For this review, take the finished solid that the model builds, in its own axes (mm). Face numbers are marked on the shaded views. A direction names the side the tool comes from. Round coordinates to 2 decimals unless told otherwise and drop trailing zeros. Write each loop counter-clockwise with the first axis right and the second up, starting at its lowest first coordinate (ties: lowest second). Pieces come first, ordered by that corner, then holes. Notation, with made-up numbers: (46.5, -32.5) -> (67.5, -32.5) arc R4 cw to (67.5, -26.5) -> close; hole circle Ø9 at (9.25, -33.75). An arc over 180 degrees is marked (long way). Write each question's results on one line, items separated by ' | '. Start each with the question number.
Item 1: Tool access review of the marked faces 1, 2, 3 and 4: name each direction out of +Z, -Z, +X, -X, +Y, -Y from which nothing blocks a thin tool from reaching the whole face with its end or side.
Item 2: The part is to be moulded in two halves that separate along X. For the marked faces 5, 6 and 7, say which applies: +X half, -X half, draft (parallel to the pull), parting line (faces both ways), or undercut.
Item 3: To check wall thickness, follow line 1 along Z through (x, y) = (2, 20.25); line 2 along Y through (x, z) = (0, 0.3); line 3 along Y through (x, z) = (-4.25, 2). State the ranges of each line that lie inside material, in increasing order.
Item 4: Add section C-C (x = 4). State the section outline as (y, z) points.
Item 5: Add section B-B (z = -4). State the section outline as (x, y) points, plus the area to 3 significant figures.
Item 6: Clearance check with flat-ended pins moving along their axes: pin 1 (4 mm diameter, centred on y = 21.5, z = 0, fed in from -X); pin 2 (1 mm diameter, centred on x = 2.5, y = 20, fed in from -Z); pin 3 (0.8 mm diameter, centred on x = -2, y = 6, fed in from -Z); pin 4 (2 mm diameter, centred on x = 2, z = 1, fed in from -Y). State where each tip first meets the part, or that it passes through.
Item 7: Add section A-A (y = 22). State the section outline as (x, z) points.
from build123d import *

# Parameters (mm, degrees)
SKETCH3_R           = 4.65
BOSS_EXTRUDE1_DEPTH = 20
SKETCH4_R           = 1
BOSS_EXTRUDE2_DEPTH = 2.5
BOSS_EXTRUDE3_START = -2.5
BOSS_EXTRUDE3_DEPTH = 10
CIRPATTERN1_COUNT   = 4
CIRPATTERN1_ANGLE   = 45


with BuildPart() as part:
    # Sketch3 → Boss-Extrude1 (new body)
    with BuildSketch(Plane(origin=(0, 0, 0), x_dir=(1, 0, 0), z_dir=(0, 1, 0))):
        with Locations(Location((0, 0, 0), (0, 0, 270))):
            Circle(SKETCH3_R)
    extrude(amount=BOSS_EXTRUDE1_DEPTH)

    # Sketch4 → Boss-Extrude2 (add, symmetric)
    with BuildSketch(Plane.XY):
        with BuildLine():
            Line((3, 20), (-3, 20))
            Line((-3, 20), (-3, 25))
            ThreePointArc((-3, 25), (0, 28), (3, 25))
            Line((3, 25), (3, 20))
        make_face()
        with Locations((0, 25)):
            Circle(SKETCH4_R, mode=Mode.SUBTRACT)
    extrude(amount=BOSS_EXTRUDE2_DEPTH, both=True)

    # Sketch5 → Boss-Extrude3 (add)
    with BuildSketch(Plane.XZ.offset(BOSS_EXTRUDE3_START)):
        Polygon((-5, 0), (-2.5, -4.330127019), (2.5, -4.330127019), (5, 0), (2.5, 4.330127019), (-2.5, 4.330127019), align=None)
    boss_extrude3 = extrude(amount=-BOSS_EXTRUDE3_DEPTH)

    # CirPattern1: Boss-Extrude3 ×4 about axis
    cirpattern1_axis = Axis((0, 0, 0), (0, -1, 0))
    for i in range(1, CIRPATTERN1_COUNT):
        add(boss_extrude3.rotate(cirpattern1_axis, i * CIRPATTERN1_ANGLE / (CIRPATTERN1_COUNT - 1)))


solid = part.part
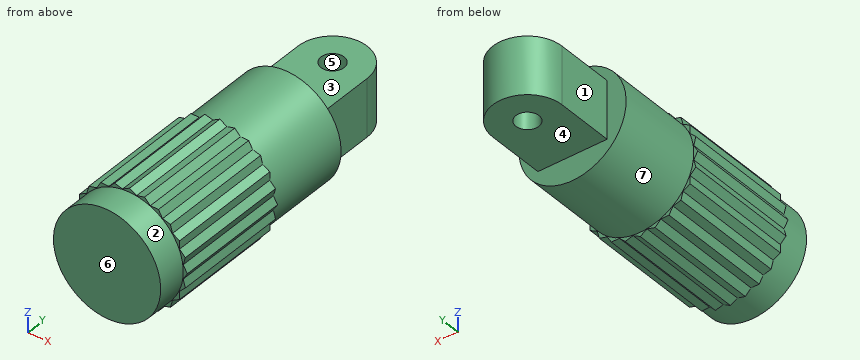
Responses:
1) face 1: +Z, -Z, -X, +Y | face 2: -Y | face 3: +Z, +X, -X, +Y | face 4: -Z, +X, -X, +Y
2) face 5: undercut | face 6: draft | face 7: parting line
3) line 1: z = -2.5 to 2.5 | line 2: y = 0 to 24, 26 to 28 | line 3: y = 2.5 to 12.5
4) outline: (0, -2.37) -> (2.5, -2.37) -> (2.5, -2.69) -> (12.5, -2.69) -> (12.5, -2.37) -> (20, -2.37) -> (20, 2.37) -> (12.5, 2.37) -> (12.5, 2.69) -> (2.5, 2.69) -> (2.5, 2.37) -> (0, 2.37) -> close
5) outline: (-2.69, 2.5) -> (-2.37, 2.5) -> (-2.37, 0) -> (2.37, 0) -> (2.37, 2.5) -> (2.69, 2.5) -> (2.69, 12.5) -> (2.37, 12.5) -> (2.37, 20) -> (-2.37, 20) -> (-2.37, 12.5) -> (-2.69, 12.5) -> close | area: 101 mm^2
6) pin 1: stops at x = -4.65 | pin 2: stops at z = -4.2 | pin 3: stops at z = -4.52 | pin 4: stops at y = 0
7) outline: (-3, -2.5) -> (3, -2.5) -> (3, 2.5) -> (-3, 2.5) -> close
